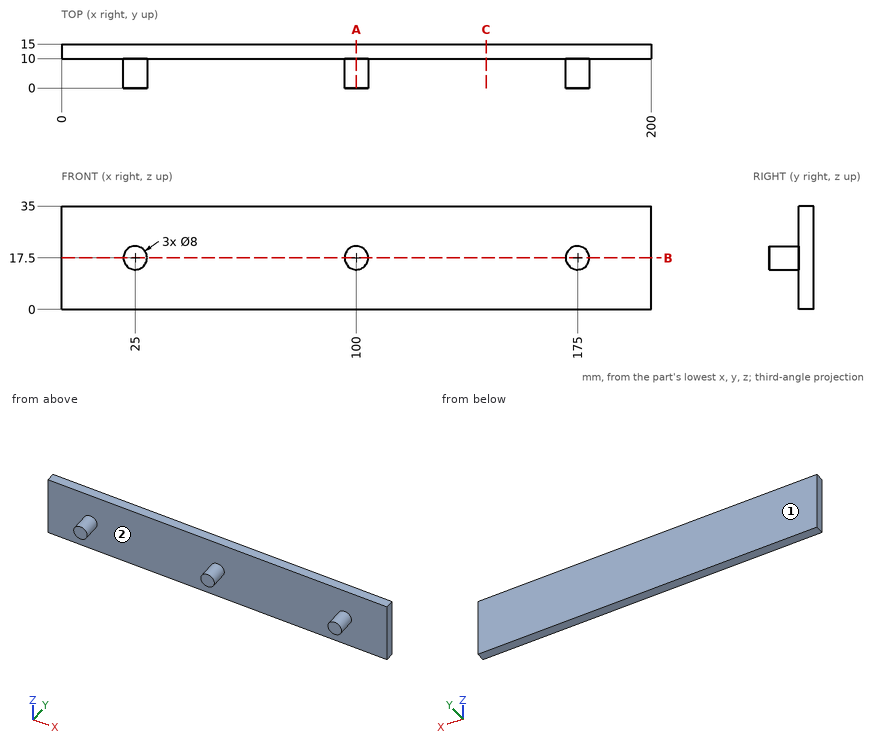
Job drawing, mm, ordinate dimensions from the low corner. One solid piece. Coordinates: 2 decimals unless noted, no trailing zeros. Order: outer loops, then holes, each group sorted by start corner. A loop starts at its lowest first (then second) coordinate and runs counter-clockwise, first axis right, second up. Notation, with made-up numbers: (-10, 72.5) -> (45, 72.5) arc R26 cw to (45, 99.5) -> close; hole circle Ø8 at (-36.75, 55). An arc over 180 degrees is marked (long way). Return JSON: item names as keys, results as strings. Group by question number.
Item 1: Flat gauge pins, fed straight in: P1, Ø6, axis at x = 179.5, z = 3.5, coming from the -Y side; P2, Ø1, axis at y = 8.5, z = 18, coming from the -X side; P3, Ø8, axis at y = 6.5, z = 18.5, coming from the +X side. Where does each tip first touch, or does it go through?
Item 2: Saw through at C-C on x = 144. Write the cut outline in (y, z), then the cut area to 3 significant figures.
Item 3: Saw through at B-B on z = 17.5. Write the cut outline in (x, y), then the cut area to 3 significant figures.
Item 4: Saw through at A-A on x = 100. Write the cut outline in (y, z), then the cut area to 3 significant figures.
Item 5: Pull direction X, two halves, no side cores. Call the marked faces 1 and 2: pulls with the +X half, pulls with the -X half, needs draft (parallel to the pull), parting line crosses it, or undercut.
Item 6: Wall check: line 1 along Y through (x, z) = (156, 7.5); line 2 along Z through (x, y) = (24.5, 0.5); line 3 along X through (y, z) = (2.25, 21). Give the ranges that are in metal, low to high. Write a range as [from, to].
Values found:
{
 "1": {"P1": "stops at y = 10", "P2": "stops at x = 21", "P3": "stops at x = 200"},
 "2": {"outline": "(10, 0) -> (15, 0) -> (15, 35) -> (10, 35) -> close", "area": "175 mm2"},
 "3": {"outline": "(0, 10) -> (21, 10) -> (21, 0) -> (29, 0) -> (29, 10) -> (96, 10) -> (96, 0) -> (104, 0) -> (104, 10) -> (171, 10) -> (171, 0) -> (179, 0) -> (179, 10) -> (200, 10) -> (200, 15) -> (0, 15) -> close", "area": "1,240 mm2"},
 "4": {"outline": "(0, 13.5) -> (10, 13.5) -> (10, 0) -> (15, 0) -> (15, 35) -> (10, 35) -> (10, 21.5) -> (0, 21.5) -> close", "area": "255 mm2"},
 "5": {"face 1": "needs draft", "face 2": "undercut"},
 "6": {"line 1": "y = [10, 15]", "line 2": "z = [13.53, 21.47]", "line 3": "x = [23.06, 26.94], [98.06, 101.94], [173.06, 176.94]"}
}
